Solid Edge part; units mm, degrees
sketch "Sketch1" plane through (0, 0, 0) normal (0, 0, 1) x (1, 0, 0)
  circle A0 centre (-90, 0.1981) radius 15
  line L0 (-150, 50) -> (150, 50)
  line L1 (150, 50) -> (150, -50)
  line L2 (150, -50) -> (-150, -50)
  line L3 (-150, -50) -> (-150, 50)
  dimension "D1" = 150
  dimension "D2" = 150
extrude "Protrusion1" add sketch "Sketch1" along normal blind 20
sketch "Sketch2" plane through (150, 0, 10) normal (1, 0, 0) x (0, 1, 0)
  circle A0 centre (0, 55) radius 25
  line L0 (-50, 10) -> (50, 10)
  line L1 (50, 10) -> (50, 90)
  line L2 (50, 90) -> (-50, 90)
  line L3 (-50, 90) -> (-50, 10)
  dimension "D1" = 50
extrude "ExtrudedProtrusion_2" add sketch "Sketch2" against normal blind 130
Input: part model. Units: mm. Frame: model coordinates. A direction names the side the tool comes from. Round coordinates to 2 decimals unless told otherwise and drop trailing zeros. Loops run counter-clockwise (first coordinate to the right, second up) from the corner with the lowest first, then second, coordinate; pieces in that order, holes last.
1) Pin query (flat end, axial travel): pin 1 (4 mm diameter, centred on y = 1.5, z = 38.5, fed in from -X); pin 2 (24 mm diameter, centred on x = -90, y = 0.2, fed in from -Z); pin 3 (3 mm diameter, centred on x = -10, y = -8, fed in from +Z). Return the tip coordinate at first contact, or that it passes through.
Ans:
pin 1: stops at x = 20
pin 2: passes through
pin 3: stops at z = 20
2) Set-up query: faces 5 (the flat face through (150, 1, 38)), 6 (the flat face through (-64, 1, 20)). Return all of +Z, -Z, +X, -X, +Y, -Y with unobstructed straight access to the full face (end or side cutting, diameter ignored); none if empty.
Ans:
face 5: +Z, -Z, +X, +Y, -Y
face 6: +Z, -X, +Y, -Y
3) Section query B-B on y = -20. Return the cut outline in (x, z).
Ans:
outline: (-150, 0) - (150, 0) - (150, 50) - (20, 50) - (20, 20) - (-150, 20) - close; (20, 80) - (150, 80) - (150, 100) - (20, 100) - close
4) Section query A-A on x = -90. Return the cut outline in (y, z).
Ans:
outline: (-50, 0) - (-14.8, 0) - (-14.8, 20) - (-50, 20) - close; (15.2, 0) - (50, 0) - (50, 20) - (15.2, 20) - close
5) Material intervals for line 1 (Z direction, x = 118, y = 0); line 2 (Y direction, x = -90, z = 8.25); line 3 (X direction, y = 18.5, z = 31.5), sorted ascending.
Ans:
line 1: z = 0 to 40, 90 to 100
line 2: y = -50 to -14.8, 15.2 to 50
line 3: x = 20 to 150
6) Section query C-C on z = 80. Return the cut outline in (x, y).
Ans:
outline: (20, -50) - (150, -50) - (150, -20) - (20, -20) - close; (20, 20) - (150, 20) - (150, 50) - (20, 50) - close
7) Section query D-D on x = 95.5. Return the cut outline in (y, z), plus the area to 3 significant figures.
Ans:
outline: (-50, 0) - (50, 0) - (50, 100) - (-50, 100) - close; hole circle Ø50 at (0, 65)
area: 8,040 mm2
8) Pull-direction query (Z, two-part tool) for faces 1 (the flat face through (2, 1, 0)), 2 (the flat face through (20, -12, 42)), 3 (the cylindrical face through (85.91, -5.42, 40.594)), 4 (the flat face through (86, 1, 100)); classes: released by +Z, released by -Z, zero draft, split by the parting line, or undercut.
Ans:
face 1: released by -Z
face 2: zero draft
face 3: undercut
face 4: released by +Z
